Autodesk Inventor part; units mm, degrees
ref_plane "YZ Plane" through (0, 0, 0) normal (1, 0, 0) x (0, 1, 0)
ref_plane "XZ Plane" through (0, 0, 0) normal (0, 1, 0) x (-1, 0, 0)
ref_plane "XY Plane" through (0, 0, 0) normal (0, 0, 1) x (1, 0, 0)
sketch "Sketch1" plane through (0, 0, 0) normal (0, 0, 1) x (1, 0, 0)
  circle A0 centre (106.5872, -122.9172) radius 2.5
  circle A1 centre (106.5872, -122.9172) radius 25.4
  line L0 (81.1872, -122.9172) -> (131.9872, -122.9172)
  line L1 (131.9872, -122.9172) -> (131.9872, 16.7828)
  line L2 (131.9872, 16.7828) -> (81.1872, 16.7828)
  line L3 (81.1872, 16.7828) -> (81.1872, -122.9172)
  circle A2 centre (106.5872, -122.9172) radius 11.5
  point P0 (0, 0)
  point P1 (106.5872, -148.3172)
  dimension "d0" = 50.8
  dimension "d1" = 139.7
  dimension "d4" = 23
  dimension "d9" = 50.8
extrude "Extrusion1" add sketch "Sketch1" against normal blind 6.35 contours L0 A0 | L0 A2 A0 | A0 L0 A2 | A2 L0 A1 | L0 A1 A2 | A1 L3 L2 L1 picked at (105.8251, -122.3305)
sketch "Sketch2" plane through (0, 0, -6.35) normal (0, 0, -1) x (-1, 0, 0)
  arc A0 (-131.9872, -122.9172) -> (-81.1872, -122.9172) centre (-106.5872, -122.9172) ccw
  circle A1 centre (-106.5872, -122.9172) radius 11.5
  point P0 (0, 0)
  dimension "d5" = 23
extrude "Extrusion2" cut sketch "Sketch2" against normal through all
sketch "Sketch3" plane through (0, 0, 0) normal (0, 0, 1) x (1, 0, 0)
  circle A0 centre (106.5872, -122.9172) radius 11.5
  arc A1 (81.1872, -122.9172) -> (131.9872, -122.9172) centre (106.5872, -122.9172) ccw
  line L0 (131.9872, 16.7828) -> (131.9872, -122.9172)
  line L1 (81.1872, 16.7828) -> (131.9872, 16.7828)
  line L2 (81.1872, -122.9172) -> (81.1872, 16.7828)
  circle A2 centre (122.0872, -107.4172) radius 2
  circle A3 centre (91.0872, -107.4172) radius 2
  circle A4 centre (122.0872, -138.4172) radius 2
  circle A5 centre (91.0872, -138.4172) radius 2
  point P0 (0, 0)
properties part number "tiltColumnStepperSide"
Can you work these out from the model? Positions are in its coordinate system, mm. Round coordinates to 2 decimals unless told otherwise and drop trailing zeros. Loops run counter-clockwise (first coordinate to the right, second up) from the corner with the lowest first, then second, coordinate; pieces in that order, holes last. Notation, with made-up numbers: (-30, 6.5) -> (-4, 6.5) arc R19 ccw to (-4, 23.5) -> close; hole circle Ø1 at (87.25, 56.25). An arc over 180 degrees is marked (long way). Answer in a Markdown table with one row per item.
Item 1: We'd pull the mould along X, two halves only. Please class faces 1 (the flat face through (131.987, -54, -3)), 2 (the cylindrical face through (115.06, -115.14, -3.22)), 3 (the flat face through (106, -65, 0)): released by +X, released by -X, zero draft, split by the parting line, or undercut.
Answer block:
| item | result |
|---|---|
| face 1 | released by +X |
| face 2 | undercut |
| face 3 | zero draft |
Item 2: Suppose I cut it at C-C, the plane x = 89. List the corners of the cut face in (y, z) for me.
Answer block:
| item | result |
|---|---|
| outline | (-141.24, -6.35) -> (16.78, -6.35) -> (16.78, 0) -> (-141.24, 0) -> close |
Item 3: Suppose I cut it at B-B, the plane x = 97.5. List the corners of the cut face in (y, z) for me.
Answer block:
| item | result |
|---|---|
| outline | (-146.64, -6.35) -> (-129.97, -6.35) -> (-129.97, 0) -> (-146.64, 0) -> close; (-115.87, -6.35) -> (16.78, -6.35) -> (16.78, 0) -> (-115.87, 0) -> close |
Item 4: If I drill on probe 1 along Y at (x, z) = (113, -2.25); probe 2 along Y at (x, z) = (99, -5.25); probe 3 along Y at (x, z) = (123.5, -2.25), over which ranges is the centre line in solid material (lowest first)?
Answer block:
| item | result |
|---|---|
| probe 1 | -147.49 to -132.46, -113.37 to 16.78 |
| probe 2 | -147.16 to -131.56, -114.28 to 16.78 |
| probe 3 | -141.87 to 16.78 |
Item 5: Suppose I cut it at A-A, the plane z = -5. List the corners of the cut face in (x, y) for me, plus the area to 3 significant figures.
Answer block:
| item | result |
|---|---|
| outline | (81.19, -122.92) arc R25.4 ccw to (131.99, -122.92) -> (131.99, 16.78) -> (81.19, 16.78) -> close; hole circle Ø23 at (106.59, -122.92) |
| area | 7,690 mm² |
